Design review of the part shown in the three views and the two pictorial views. Dimensions are in mm from the part's minimum x, y and z. Give positions to 0.01 mm unless a question says otherwise; leave off trailing zeros. Order: outer loops, then holes, each group sorted by start corner. A loop starts at its lowest first (then second) coordinate and runs counter-clockwise, first axis right, second up.
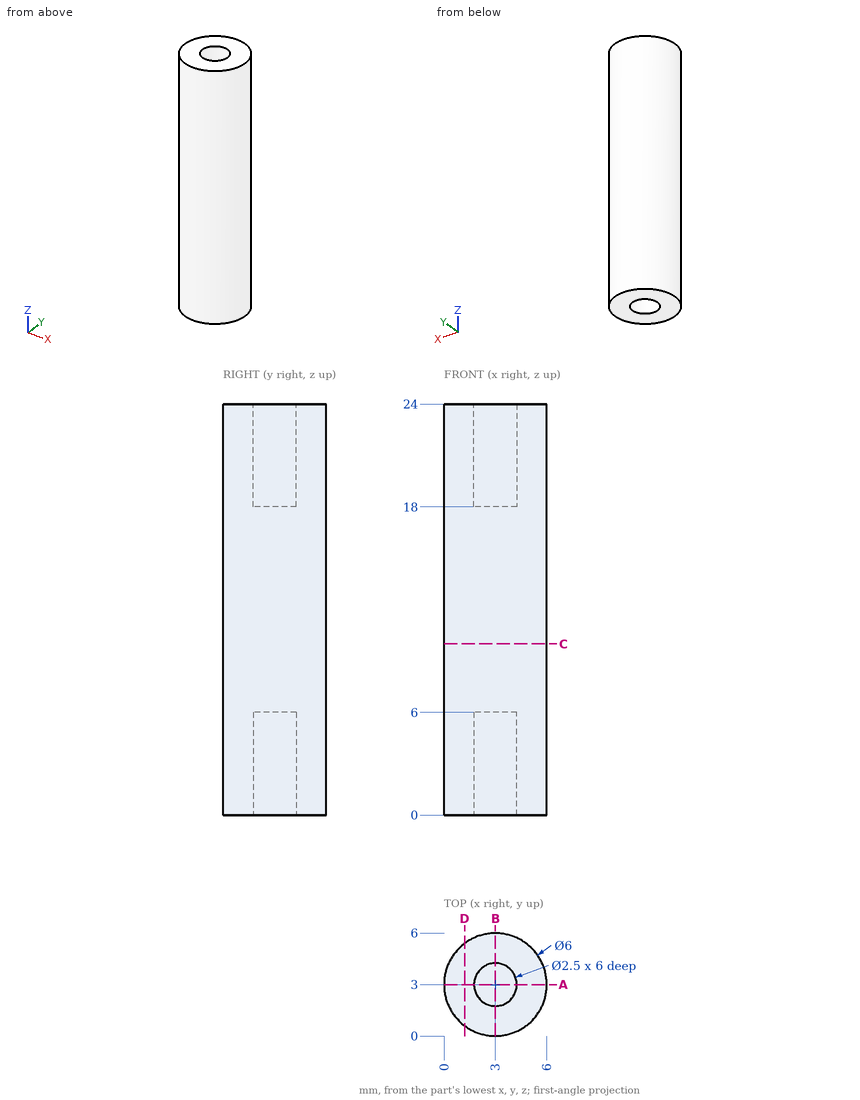
Item 1: Take a section at A-A (y = 3). Give the boundary of the cut face in (x, z), and give its area (3 significant figures).
Values found:
outline: (0, 0) - (1.75, 0) - (1.75, 6) - (4.25, 6) - (4.25, 0) - (6, 0) - (6, 24) - (4.25, 24) - (4.25, 18) - (1.75, 18) - (1.75, 24) - (0, 24) - close
area: 114 mm2
Item 2: Take a section at D-D (x = 1.2). Give the boundary of the cut face in (y, z), and give its area (3 significant figures).
Values found:
outline: (0.6, 0) - (5.4, 0) - (5.4, 24) - (0.6, 24) - close
area: 115 mm2
Item 3: Clearance check with flat-ended pins moving along their axes: pin 1 Ø2 at (x, z) = (1, 2.5) entering from -Y; pin 2 Ø1 at (y, z) = (1, 6) entering from +X; pin 3 Ø1.2 at (x, y) = (3, 3) entering from -Z. State where each tip first meets the part, or that it passes through.
Values found:
pin 1: stops at y = 0.17
pin 2: stops at x = 5.6
pin 3: stops at z = 6
Item 4: For line 1 (Y direction, x = 3, z = 21.55); line 2 (Z direction, x = 2.75, y = 3.8); line 3 (Y direction, x = 3.85, z = 22), list the stretches that pass through material, from the lowest coordinate up.
Values found:
line 1: y = 0 to 1.75, 4.25 to 6
line 2: z = 6 to 18
line 3: y = 0.12 to 2.08, 3.92 to 5.88
Item 5: Take a section at C-C (z = 10). Give the boundary of the cut face in (x, y).
Values found:
outline: circle Ø6 at (3, 3)
